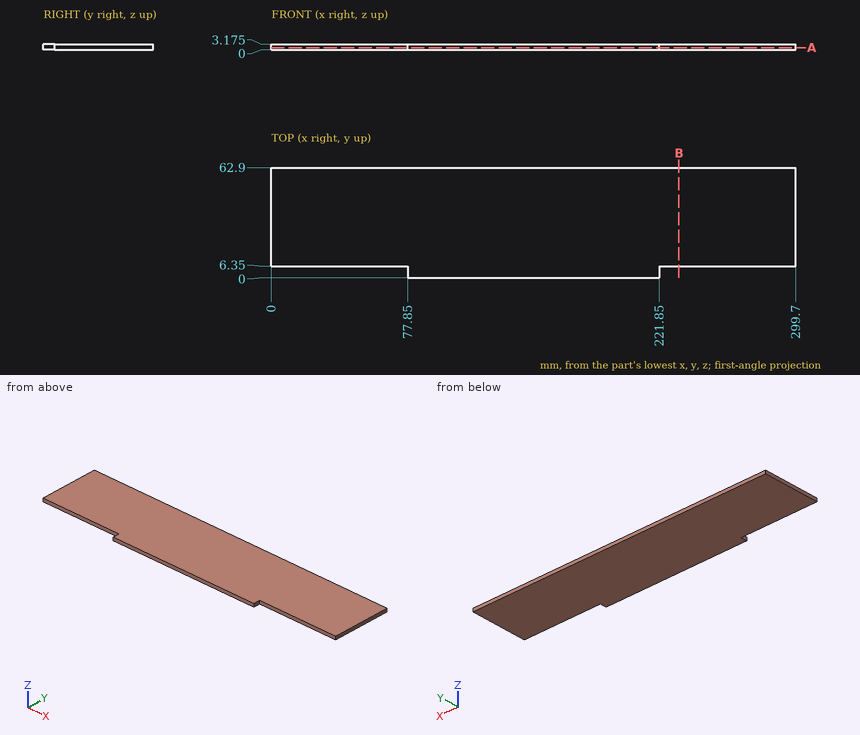
Study the drawing (mm; zero at the part's minimum x, y, z) and answer. Give positions to 0.01 mm unless a question says otherwise; leave off trailing zeros. Order: outer loops, then holes, each group sorted by start corner. A loop starts at its lowest first (then second) coordinate and runs counter-clockwise, first axis right, second up. Notation, with made-up numbers: (11, -1) - (61, -1) arc R12 cw to (61, 5) - close; hole circle Ø4 at (-9.75, 89.5). An arc over 180 degrees is marked (long way). Answer in a Markdown table with one row per item. Add a question column.
Q1. Find the intervals of material crossed by line 1 along Y through (x, z) = (45, 2.95), in increasing order. Write a range as [from, to].
Q2. The part is cut by section A-A (z = 1.1). Determine the outline of the cut face in (x, y), then the cut area to 3 significant figures.
Q3. Given P1, Ø1, axis at y = 2, z = 2, coming from the -X side; P2, Ø1.6, axis at y = 3, z = 1, coming from the +X side; P3, Ø1, axis at x = 242, z = 1, coming from the -Y side, each flat-ended and moving along its own axis, determine where each tip first touches the part or whether it passes through.
Q4. The part is cut by section B-B (x = 233). Determine the outline of the cut face in (y, z) (3 decimals).
Determined:
| question | item | result |
|---|---|---|
| 1 | line 1 | y = [6.35, 62.9] |
| 2 | outline | (0, 6.35) - (77.85, 6.35) - (77.85, 0) - (221.85, 0) - (221.85, 6.35) - (299.7, 6.35) - (299.7, 62.9) - (0, 62.9) - close |
| 2 | area | 17,900 mm² |
| 3 | P1 | stops at x = 77.85 |
| 3 | P2 | stops at x = 221.85 |
| 3 | P3 | stops at y = 6.35 |
| 4 | outline | (6.35, 0) - (62.9, 0) - (62.9, 3.175) - (6.35, 3.175) - close |
